```python
from build123d import *

# Parameters (mm, degrees)
SALIENTE_EXTRUIR1_DEPTH = 1
CROQUIS3_R              = 4.875
CORTAR_EXTRUIR1_DEPTH   = 0.2
CROQUIS4_R              = 0.9
CROQUIS4_R_2            = 0.8999999999999994
SALIENTE_EXTRUIR2_DEPTH = 3.4
CHAFL_N1_SIZE           = 0.4
CROQUIS5_R              = 0.8999999999999995
CROQUIS5_R_2            = 0.9000000000000004
CORTAR_EXTRUIR2_DEPTH   = 2.4
CORTAR_EXTRUIR3_START   = -0.35
CORTAR_EXTRUIR3_DEPTH   = 0.35


with BuildPart() as part:
    # Croquis1 → Saliente-Extruir1 (new body)
    with BuildSketch(Plane(origin=(0, 0, 0), x_dir=(1, 0, 0), z_dir=(0, 1, 0))):
        with BuildLine():
            Line((6.000000000184592, 6.000000000000001), (0.6000000001845911, 6.0000000000897735))
            Line((0.6000000001845911, 6.0000000000897735), (0.600000000184591, 5.250000000089774))
            Line((0.600000000184591, 5.250000000089774), (-0.5999999998154079, 5.250000000089775))
            Line((-0.5999999998154079, 5.250000000089775), (-0.5999999998154087, 6.000000000109725))
            Line((-0.5999999998154087, 6.000000000109725), (-5.999999999815408, 6.0000000001995))
            ThreePointArc((-5.999999999815408, 6.0000000001995), (-8.349999999490638, 1.358977e-10), (-6, -6.000000000000001))
            Line((-6, -6.000000000000001), (-0.6, -6.000000000089775))
            Line((-0.6, -6.000000000089775), (-0.6, -5.250000000109726))
            Line((-0.6, -5.250000000109726), (0.6, -5.250000000109726))
            Line((0.6, -5.250000000109726), (0.6000000000000001, -6.000000000109724))
            Line((0.6000000000000001, -6.000000000109724), (6.000000000000001, -6.000000000199499))
            ThreePointArc((6.000000000000001, -6.000000000199499), (8.349999999490638, -1.3589858e-10), (6.000000000184592, 6.000000000000001))
        make_face()
    extrude(amount=SALIENTE_EXTRUIR1_DEPTH)

    # Croquis3 → Cortar-Extruir1 (cut)
    with BuildSketch(Plane(origin=(0, 1, 0), x_dir=(1, 0, 0), z_dir=(0, 1, 0))):
        with Locations(Location((0, 0, 0), (0, 0, 270))):
            Circle(CROQUIS3_R)
    extrude(amount=-CORTAR_EXTRUIR1_DEPTH, mode=Mode.SUBTRACT)

    # Croquis4 → Saliente-Extruir2 (add)
    with BuildSketch(Plane.XZ):
        with Locations(Location((0, 0, 0), (0, 0, 270))):
            Circle(CROQUIS4_R)
        with Locations(Location((-5.3500000000000005, 4.700000000000001, 0), (0, 0, 270))):
            Circle(CROQUIS4_R_2)
        with Locations(Location((-5.349999999815407, -4.700000000199502, 0), (0, 0, 270))):
            Circle(CROQUIS4_R_2)
        with Locations(Location((5.3500000000000005, 4.700000000000001, 0), (0, 0, 270))):
            Circle(CROQUIS4_R_2)
        with Locations(Location((5.3500000000000005, -4.700000000199502, 0), (0, 0, 270))):
            Circle(CROQUIS4_R_2)
        with BuildLine():
            Line((5.3500000000000005, 2.65), (5.3500000000000005, -2.65))
            Line((5.3500000000000005, -2.65), (7.9431895310497564, -2.65))
            ThreePointArc((7.9431895310497564, -2.65), (8.349999999490638, 0), (7.9431895310497564, 2.65))
            Line((7.9431895310497564, 2.65), (5.3500000000000005, 2.65))
        make_face()
        with BuildLine():
            Line((-5.349999999999999, -2.65), (-5.349999999999999, 2.65))
            Line((-5.349999999999999, 2.65), (-7.94318953102517, 2.65))
            ThreePointArc((-7.94318953102517, 2.65), (-8.349999999490638, 1.08e-15), (-7.94318953102517, -2.65))
            Line((-7.94318953102517, -2.65), (-5.349999999999999, -2.65))
        make_face()
    extrude(amount=-SALIENTE_EXTRUIR2_DEPTH)

    # Chaflán1
    chafl_n1_edges = [part.edges().sort_by_distance(p)[0] for p in [
        (2.8e-16, 3.4, 0.9),
        (-5.3500000000000005, 3.4, 5.6000000000000005),
        (5.3500000000000005, 3.4, 5.6000000000000005),
        (-5.349999999815407, 3.4, -3.8000000001995025),
        (5.3500000000000005, 3.4, -3.8000000001995025),
    ]]
    chamfer(chafl_n1_edges, length=CHAFL_N1_SIZE)

    # Croquis5 → Cortar-Extruir2 (cut)
    with BuildSketch(Plane(origin=(0, 3.4, 0), x_dir=(1, 0, 0), z_dir=(0, 1, 0))):
        with Locations(Location((-6.899999999999999, 0, 0), (0, 0, 270))):
            Circle(CROQUIS5_R)
        with Locations(Location((6.8999999999999995, 0, 0), (0, 0, 270))):
            Circle(CROQUIS5_R_2)
    extrude(amount=-CORTAR_EXTRUIR2_DEPTH, mode=Mode.SUBTRACT)

    # Croquis6 → Cortar-Extruir3 (cut)
    with BuildSketch(Plane(origin=(0, 3.4, 0), x_dir=(1, 0, 0), z_dir=(0, 1, 0)).offset(CORTAR_EXTRUIR3_START)):
        with BuildLine():
            Line((-5.349999999999999, 2.65), (-7.943189531025168, 2.6499999999999995))
            ThreePointArc((-7.943189531025168, 2.6499999999999995), (-8.349999999490636, 1.08e-15), (-7.94318953102517, -2.65))
            Line((-7.94318953102517, -2.65), (-5.349999999999999, -2.65))
            Line((-5.349999999999999, -2.65), (-5.349999999999999, 2.65))
        make_face()
        with BuildLine():
            Line((5.3500000000000005, -2.65), (7.9431895310497564, -2.6499999999999995))
            ThreePointArc((7.9431895310497564, -2.6499999999999995), (8.349999999490638, 4.9e-16), (7.9431895310497564, 2.65))
            Line((7.9431895310497564, 2.65), (5.3500000000000005, 2.65))
            Line((5.3500000000000005, 2.65), (5.3500000000000005, -2.65))
        make_face()
    extrude(amount=CORTAR_EXTRUIR3_DEPTH, mode=Mode.SUBTRACT)


solid = part.part
```
Check sheet for the modelled part. Datum: model origin and axes. Units: mm. A direction names the side the tool comes from. Coordinates: 2 decimals unless noted, no trailing zeros. Write each loop counter-clockwise with the first axis right and the second up, starting at its lowest first coordinate (ties: lowest second). Pieces come first, ordered by that corner, then holes. Notation, with made-up numbers: (42, -4.75) - (47, -4.75) arc R20 ccw to (47, 5.25) - close; hole circle Ø3 at (-22, 13). An arc over 180 degrees is marked (long way). One line per question, with ' | ' between items.
Item 1: Sectioned sample at D-D on x = 6.9. Record the boundary of the cut face in (y, z).
Determined:
outline: (0, -4.85) - (1, -4.85) - (1, -2.65) - (3.05, -2.65) - (3.05, -0.9) - (1, -0.9) - (1, 0.9) - (3.05, 0.9) - (3.05, 2.65) - (1, 2.65) - (1, 4.85) - (0, 4.85) - close
Item 2: Sectioned sample at A-A on y = 1.5. Give the number of separate pieces and of enclosed holes in the cut face, plus the area to 3 significant figures.
Determined:
separate pieces: 7 | enclosed holes: 2 | area: 38.0 mm2
Item 3: Access from +Z, -Z, +X, -X, +Y, -Y to the whole of each face (thin tool, end or side, straight path). Record for faces 1 (the face through (6, 3.05, -1)), 2 (the face through (0, 0.5, 5.25)), 3 (the face through (0, 0, 0)), 4 (the face through (5.4, 3.4, 4.7)), 5 (the face through (4.471, 1.986, -4.505)).
Determined:
face 1: +X, +Y | face 2: +Z, +Y, -Y | face 3: +Z, -Z, +X, -X, -Y | face 4: +Z, -Z, +X, -X, +Y | face 5: +Y
Item 4: Sectioned sample at C-C on y = 0.55. Record the boundary of the cut face in (x, z).
Determined:
outline: (-6, -6) - (-0.6, -6) - (-0.6, -5.25) - (0.6, -5.25) - (0.6, -6) - (6, -6) arc R8.83 ccw to (6, 6) - (0.6, 6) - (0.6, 5.25) - (-0.6, 5.25) - (-0.6, 6) - (-6, 6) arc R8.83 ccw to start
Item 5: Mould release check, pull along X, two halves, no side actions. Record for faces 6 (the face through (-8.35, 1.16, -0.09)), 7 (the face through (7, 1, 0)), 8 (the face through (3.3, 0.5, -6)): pulls with the +X half, pulls with the -X half, needs draft (parallel to the pull), parting line crosses it, or undercut.
Determined:
face 6: pulls with the -X half | face 7: undercut | face 8: needs draft
Item 6: Gauge pin test, flat ends, axial feed: P1, Ø1, axis at y = 2, z = 4, coming from the -X side; P2, Ø1, axis at x = -6, y = 2, coming from the -Z side; P3, Ø0.8, axis at y = 0.5, z = -5.5, coming from the -X side. Record the tip position at first contact, or that the pin passes through.
Determined:
P1: stops at x = -6.23 | P2: stops at z = -5.59 | P3: stops at x = -6.73
Item 7: Thickness scan on line 1 (X direction, y = 1.75, z = 0); line 2 (Y direction, x = -0.25, z = -4.25); line 3 (Z direction, x = 0.25, y = 0.45). Record the ranges inside material, lowest first. Write a range as [from, to].
Determined:
line 1: x = [-8.35, -7.8], [-6, -5.35], [-0.9, 0.9], [5.35, 6], [7.8, 8.35] | line 2: y = [0, 0.8] | line 3: z = [-5.25, 5.25]
Item 8: Sectioned sample at B-B on z = 0. Record the boundary of the cut face in (x, y) (3 decimals).
Determined:
outline: (-8.35, 0) - (8.35, 0) - (8.35, 3.05) - (7.8, 3.05) - (7.8, 1) - (6, 1) - (6, 3.05) - (5.35, 3.05) - (5.35, 1) - (4.875, 1) - (4.875, 0.8) - (0.9, 0.8) - (0.9, 3) - (0.5, 3.4) - (-0.5, 3.4) - (-0.9, 3) - (-0.9, 0.8) - (-4.875, 0.8) - (-4.875, 1) - (-5.35, 1) - (-5.35, 3.05) - (-6, 3.05) - (-6, 1) - (-7.8, 1) - (-7.8, 3.05) - (-8.35, 3.05) - close
